Autodesk Inventor part; units mm, degrees
ref_plane "YZ Plane" through (0, 0, 0) normal (1, 0, 0) x (0, 1, 0)
ref_plane "XZ Plane" through (0, 0, 0) normal (0, 1, 0) x (-1, 0, 0)
ref_plane "XY Plane" through (0, 0, 0) normal (0, 0, 1) x (1, 0, 0)
sketch "Profile" plane through (0, 0, 0) normal (0, 0, 1) x (1, 0, 0)
  line L0 (0, 19.34) -> (0, -4.04)
  line L1 (-9.52, 0) -> (9.52, 0)
  line L2 (-6.8, 3) -> (-3.1, -0.7)
  line L3 (-3.1, -0.7) -> (3.1, -0.7)
  line L4 (3.1, -0.7) -> (6.8, 3)
  line L5 (6.8, 3) -> (4, 3)
  line L6 (4, 3) -> (4, 6)
  line L7 (-6.8, 3) -> (-4, 3)
  line L8 (-4, 3) -> (-4, 6)
  line L9 (-4, 6) -> (4, 6)
  line L10 (-2, 6) -> (-2, 16)
  line L11 (-2, 16) -> (2, 16)
  line L12 (2, 16) -> (2, 6)
  point P0 (0, 0)
  dimension "d0" = 13.6
  dimension "d1" = 3
  dimension "d2" = 45
  dimension "d3" = 3.7
  dimension "d4" = 3
  dimension "d5" = 8
  dimension "d6" = 4
  dimension "d7" = 10
extrude "Body" add sketch "Profile" along normal mid plane 2
sketch "RotateSketch" plane through (0, 0, 0) normal (1, 0, 0) x (0, 1, 0)
  line L0 (0, 11.2) -> (0, -11.2)
  circle A0 centre (0, 0) radius 5.25
  circle A1 centre (0, 0) radius 8
  point P0 (0, 8)
  point P1 (0, 5.25)
  point P2 (0, -5.25)
  point P3 (0, -8)
  dimension "d10" = 10.5
  dimension "d11" = 16
extrude "RotateEdge" cut sketch "RotateSketch" along normal blind 2 from surface at 2 contours A1 L0 A0 picked at (3.9108, -5.8557)
mirror "Mirror" about plane through (0, 0, 0) normal (1, 0, 0) of "RotateEdge"
properties part number "SwitchLeverUnit_Lever"
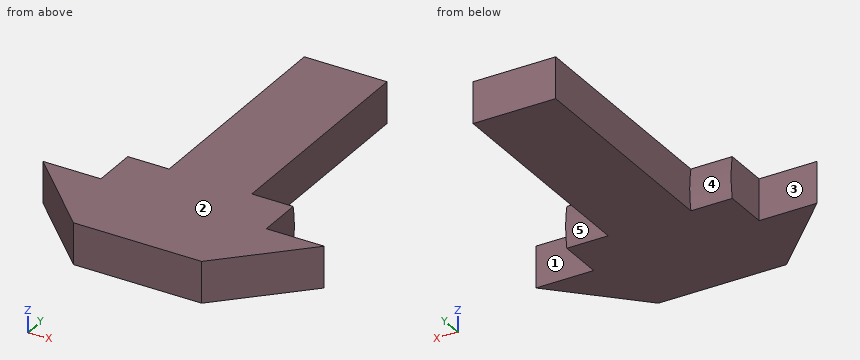
Can you work these out from the model? Positions are in its coordinate system, mm. Face numbers are marked on the shaded views. A direction names the side the tool comes from. Give positions to 0.01 mm unless a question says otherwise; leave off trailing zeros. Loops run counter-clockwise (first coordinate to the right, second up) from the corner with the lowest first, then second, coordinate; pieces in that order, holes last. Notation, with made-up numbers: M 16.25,-26.5 L 48.25,-26.5 A22 ccw 48.25,-3.5 Z; hole C 2.5,61 d10. An arc over 180 degrees is marked long. Use one line per item in the form item = value. Start each with the question number.
(1) I want a section at B-B, the plane x = 3.75. Write out the boundary of the cut face in (y, z), and give its area (3 significant figures).
(2) I want a section at A-A, the plane z = -0.05. Write out the boundary of the cut face in (x, y).
(3) I want a section at C-C, the plane y = 13. Write out the boundary of the cut face in (x, z).
(4) I'm going to push flat-ended pins straight in: P1, Ø1, axis at y = 4, z = 0, coming from the -X side; P2, Ø1, axis at y = 4, z = 0, coming from the +X side; P3, Ø0.6, axis at y = 9.5, z = 0, coming from the -X side; P4, Ø4, axis at x = -4.5, y = 10, coming from the +Z side. Where does each tip first touch, or does it pass through?
(5) Please list where these lines run through material, in increasing order: line 1 (X direction, y = 10.75, z = 0.75); line 2 (X direction, y = 3.75, z = 0.8); line 3 (Y direction, x = 2.25, z = -0.1).
(6) On a 3-axis mill with a long thin cutter (end or side, diameter ignored), from which of +Z, -Z, +X, -X, +Y, -Y can I reach the whole of each face in a straight line? I mean the marked faces 1, 2, 3, 4 and 5. Say none if no direction works.
Worked out:
q1.outline = M -0.05,-1 L 5.15,-1 A5.25 ccw 5.15,1 L -0.05,1 Z
q1.area = 10.5 mm²
q2.outline = M -6.8,3 L -3.1,-0.7 L 3.1,-0.7 L 6.8,3 L 4,3 L 4,5.25 L 2,5.25 L 2,16 L -2,16 L -2,5.25 L -4,5.25 L -4,3 Z
q3.outline = M -2,-1 L 2,-1 L 2,1 L -2,1 Z
q4.P1 = -4
q4.P2 = 4
q4.P3 = -2
q4.P4 = through
q5.line_1 = -2 to 2
q5.line_2 = -4 to 4
q5.line_3 = -0.7 to 5.25
q6.face_1 = +Z, -Z, +X, +Y
q6.face_2 = +Z, +X, -X, +Y, -Y
q6.face_3 = +Z, -Z, -X, +Y
q6.face_4 = -X, +Y
q6.face_5 = +X, +Y
